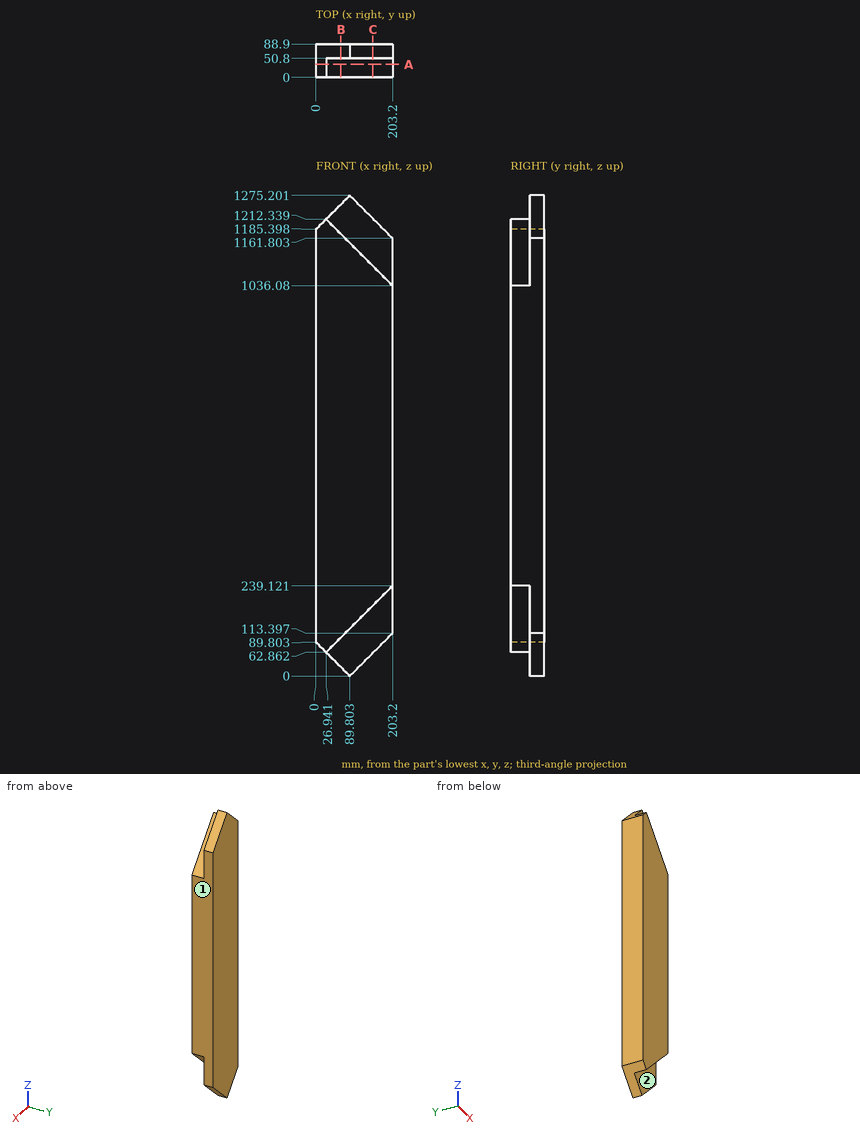
Geometry: see drawing. Coordinates: mm, zero at the bounding-box minimum. A direction names the side the tool comes from. Give positions to 0.01 mm unless a question says otherwise; leave off trailing zeros. Loops run counter-clockwise (first coordinate to the right, second up) from the corner with the lowest first, then second, coordinate; pieces in that order, holes last. Notation, with made-up numbers: (25.5, 75) -> (64.5, 75) arc R37 ccw to (64.5, 114) -> close; hole circle Ø1 at (-17.75, 79). An arc over 180 degrees is marked (long way). Put each result on its own line as item: value.
1. Set-up query: the marked faces 1 and 2. Return all of +Z, -Z, +X, -X, +Y, -Y with unobstructed straight access to the full face (end or side cutting, diameter ignored); none if empty.
Taken from the geometry:
face 1: +Z, -Z, +X, +Y, -Y
face 2: -Z, +X, -Y
2. Ray query, line 1 along Y through (x, z) = (173, 201.5); line 2 along Z through (x, y) = (184.5, 27); line 3 along Z through (x, y) = (136, 74) (1 decimal). Return the intervals inside material, ascending. Write a range as [from, to].
Taken from the geometry:
line 1: y = [50.8, 88.9]
line 2: z = [220.42, 1054.78]
line 3: z = [46.2, 1229]
3. Cut plane A-A (y = 34.5). Return the cut outline in (x, z).
Taken from the geometry:
outline: (0, 89.8) -> (26.94, 62.86) -> (203.2, 239.12) -> (203.2, 1036.08) -> (26.94, 1212.34) -> (0, 1185.4) -> close
4. Cut plane C-C (x = 151). Return the cut outline in (y, z), plus the area to 3 significant figures.
Taken from the geometry:
outline: (0, 186.92) -> (50.8, 186.92) -> (50.8, 61.2) -> (88.9, 61.2) -> (88.9, 1214) -> (50.8, 1214) -> (50.8, 1088.28) -> (0, 1088.28) -> close
area: 89,700 mm2
5. Cut plane B-B (x = 66). Return the cut outline in (y, z), plus the area to 3 significant figures.
Taken from the geometry:
outline: (0, 101.92) -> (50.8, 101.92) -> (50.8, 23.8) -> (88.9, 23.8) -> (88.9, 1251.4) -> (50.8, 1251.4) -> (50.8, 1173.28) -> (0, 1173.28) -> close
area: 101,000 mm2
6. Pin query (flat end, axial travel): P1, Ø12, axis at x = 35, y = 52.5, coming from the -Z side; P2, Ø5, axis at x = 35.5, y = 13, coming from the +Z side; P3, Ø5, axis at x = 135, y = 50.5, coming from the +Z side (1 decimal). Return the tip coordinate at first contact, or that it passes through.
Taken from the geometry:
P1: stops at z = 48.8
P2: stops at z = 1206.28
P3: stops at z = 1232.5
